from build123d import *

# Parameters (mm, degrees)
BOSS_EXTRUDE1_DEPTH = 42
SKETCH3_7_R         = 3.3
SKETCH2_6_R         = 6.3


with BuildPart() as part:
    # Sketch1 → Boss-Extrude1 (new, symmetric)
    with BuildSketch(Plane(origin=(0, 0, 0), x_dir=(1, 0, 0), z_dir=(0, 1, 0))):
        Polygon((0, 20.057673142), (0, -20.092326858), (-5, -20.092326858), (-2.895827662, 20.057673142), align=None)
    extrude(amount=BOSS_EXTRUDE1_DEPTH, both=True)

    # Loft2: read off the stored shape, not the designer's step
    # Loft2: loft between two sections, ruled curve by curve
    loft2_from = [
        Edge.make_bspline([(-6.744919191, -26.766256905, -3.934599382), (-7.072478945, -28.860904588, 2.315613069), (-6.962853556, -35.119694494, 0.223836028), (-6.635293801, -33.025046811, -6.026376424), (-6.307734047, -30.930399127, -12.276588875), (-6.417359436, -24.671609222, -10.184811834), (-6.744919191, -26.766256905, -3.934599382)], [0, 0, 0, 0, 0.5, 0.5, 0.5, 1, 1, 1, 1], 3, [1, 0.333333333, 0.333333333, 1, 0.333333333, 0.333333333, 1]),
    ]
    loft2_to = [
        Edge.make_bspline([(-3.874025978, -24.614903671, -1.39253736), (-4.42677199, -31.486205901, 9.154484851), (-4.067155817, -42.047702275, 2.292599502), (-3.514409805, -35.176400045, -8.254422709), (-2.961663793, -28.305097815, -18.801444919), (-3.321279966, -17.743601441, -11.93955957), (-3.874025978, -24.614903671, -1.39253736)], [0, 0, 0, 0, 0.5, 0.5, 0.5, 1, 1, 1, 1], 3, [1, 0.333333333, 0.333333333, 1, 0.333333333, 0.333333333, 1]),
    ]
    loft2 = Solid(Shell([*[Face.make_surface_from_curves(loft2_from[k], loft2_to[k]) for k in range(1)], Face(Wire(loft2_from)), Face(Wire(loft2_to))]))
    add(loft2)

    # Sketch3<7> → Loft3 section 0
    with BuildSketch(Plane(origin=(-6.932083318, 0, -0.363295092), x_dir=(-0.052335956242940435, 0, 0.998629534754574), z_dir=(-0.9986295347545742, 0, -0.052335956242940435))):
        with Locations((-4.623529197, 29.895651858)):
            Circle(SKETCH3_7_R)
    # Sketch2<6> → Loft3 section 1
    with BuildSketch(Plane(origin=(-3.936194713, 0, -0.206287224), x_dir=(-0.052335956242940435, 0, 0.998629534754574), z_dir=(-0.9986295347545742, 0, -0.052335956242940435))):
        with Locations((-4.623529197, 29.895651858)):
            Circle(SKETCH2_6_R)
    loft()


solid = part.part
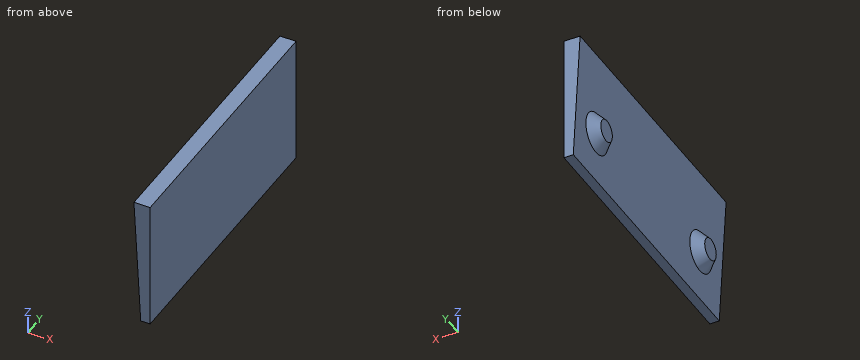
Model file for the job. Use its own axes, mm. Coordinates: 2 decimals unless noted, no trailing zeros. Order: outer loops, then holes, each group sorted by start corner. A loop starts at its lowest first (then second) coordinate and runs counter-clockwise, first axis right, second up. Notation, with made-up numbers: (-18, 40) -> (-11, 40) arc R25 ccw to (-11, 58) -> close; hole circle Ø6 at (78.25, 88). An arc over 180 degrees is marked (long way). Return JSON: item names as keys, results as strings. Group by question number.
Item 1: Wall check: line 1 along Y through (x, z) = (-5, -6); line 2 along X through (y, z) = (34, 7.5); line 3 along Y through (x, z) = (-5.75, -2.5). Give the ranges that are in metal, low to high. Write a range as [from, to].
Item 2: Saw through at B-B on z = -12. Write the cut outline in (x, y).
Item 3: Saw through at A-A on y = 15.5. Write the cut outline in (x, z), then the cut area to 3 significant figures.
Item 4: Flat gauge pins, fed straight in: P1, Ø3, axis at y = -7.5, z = -15.5, coming from the -X side; P2, Ø10, axis at y = -29.5, z = 13.5, coming from the -X side. Where does each tip first touch, or does it go through?
Values found:
{
 "1": {"line 1": "y = [-34.67, -25.12], [25.09, 34.7]", "line 2": "x = [-4.34, 0]", "line 3": "y = [-33.49, -26.31], [26.26, 33.53]"},
 "2": {"outline": "(-3.32, -42) -> (0, -42) -> (0, 42) -> (-3.32, 42) -> close"},
 "3": {"outline": "(-5, 20.09) -> (-2.9, -20.06) -> (0, -20.06) -> (0, 20.09) -> close", "area": "159 mm2"},
 "4": {"P1": "stops at x = -3.21", "P2": "stops at x = -4.92"}
}
